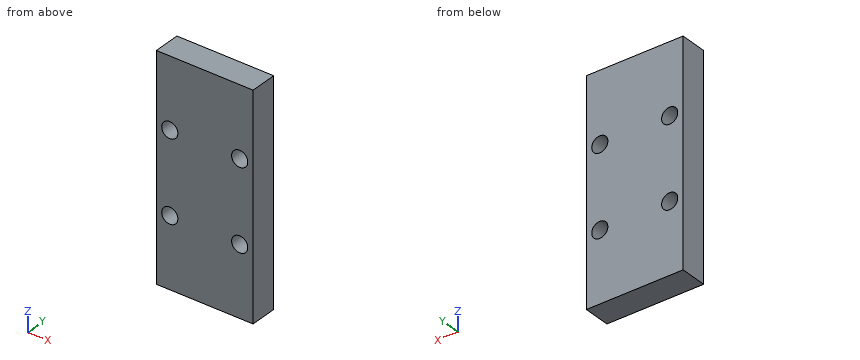
```python
from build123d import *

# Parameters (mm, degrees)
SKETCH1_W           = 9
SKETCH1_H           = 41
SKETCH1_R           = 1.5
BOSS_EXTRUDE1_DEPTH = 5


with BuildPart() as part:
    # Sketch1 → Boss-Extrude1 (new body)
    with BuildSketch(Plane(origin=(0, 0, 0), x_dir=(1, 0, 0), z_dir=(0, 1, 0))):
        with Locations((4.5, 20.5)):
            Rectangle(SKETCH1_W, SKETCH1_H)
        with Locations(Location((2.5, 13, 0), (0, 0, 270))):
            Circle(SKETCH1_R, mode=Mode.SUBTRACT)
        with Locations(Location((2.5, 28, 0), (0, 0, 270))):
            Circle(SKETCH1_R, mode=Mode.SUBTRACT)
    boss_extrude1 = extrude(amount=BOSS_EXTRUDE1_DEPTH)

    # Mirror1: Boss-Extrude1 across plane
    add(boss_extrude1.mirror(Plane(origin=(9, 5, 0), x_dir=(0, 0, 1), z_dir=(-1, 0, 0))))


solid = part.part
```
Model file for the job. Use its own axes, mm. Give positions to 0.01 mm unless a question says otherwise; leave off trailing zeros. Write each loop counter-clockwise with the first axis right and the second up, starting at its lowest first coordinate (ties: lowest second). Pieces come first, ordered by that corner, then holes. Notation, with made-up numbers: (16.5, 10.25) - (26.5, 10.25) arc R22 cw to (26.5, 18.25) - close; hole circle Ø5 at (29, 47). An arc over 180 degrees is marked (long way). One line per question, with ' | ' between items. Start each with the question number.
(1) Slice it at B-B on z = -28. Write the cut outline in (x, y).
(2) Wall check: line 1 along Z through (x, y) = (15.5, 2.65); line 2 along X through (y, z) = (2.8, -28); line 3 along Z through (x, y) = (16, 2.2). Give the ranges that are in metal, low to high. Write a range as from..to.
(3) Pin check, flat tip, straight feed: P1, Ø1.5, axis at y = 1.5, z = -33, coming from the -X side. Stop position of the tip, or through.
(4) Slice it at A-A on x = 2.5. Write the cut outline in (y, z).
(5) Slice it at C-C on y = 4.2. Write the cut outline in (x, z), plus the area to 3 significant figures.
Results below:
1) outline: (0, 0) - (1, 0) - (1, 5) - (0, 5) - close; (4, 0) - (14, 0) - (14, 5) - (4, 5) - close; (17, 0) - (18, 0) - (18, 5) - (17, 5) - close
2) line 1: -41..-29.5, -26.5..-14.5, -11.5..0 | line 2: 0..1, 4..14, 17..18 | line 3: -41..-29.41, -26.59..-14.41, -11.59..0
3) P1: x = 0
4) outline: (0, -41) - (5, -41) - (5, -29.5) - (0, -29.5) - close; (0, -26.5) - (5, -26.5) - (5, -14.5) - (0, -14.5) - close; (0, -11.5) - (5, -11.5) - (5, 0) - (0, 0) - close
5) outline: (0, -41) - (18, -41) - (18, 0) - (0, 0) - close; hole circle Ø3 at (2.5, -28); hole circle Ø3 at (2.5, -13); hole circle Ø3 at (15.5, -28); hole circle Ø3 at (15.5, -13) | area: 710 mm^2
